Can you work these out from the model? Positions are in its coordinate system, mm. A direction names the side the tool comes from. Round coordinates to 2 decimals unless told otherwise and drop trailing zeros. Loops run counter-clockwise (first coordinate to the right, second up) from the corner with the lowest first, then second, coordinate; pieces in that order, holes last. Notation, with made-up numbers: (-30, 70.25) -> (10, 70.25) arc R18 ccw to (10, 92.25) -> close; hole circle Ø3 at (-30, -24.75). An arc over 180 degrees is marked (long way). Use a Markdown table: item, result.
from build123d import *

# Parameters (mm, degrees)
BOX001_W     = 100
BOX001_H     = 15
BOX001_DEPTH = 4
BOX_W        = 100
BOX_H        = 37
BOX_DEPTH    = 10
FILLET_R     = 1


with BuildPart() as cutter:
    # Box001 → Box001 (new body)
    with BuildSketch(Plane.XY.offset(3)):
        with Locations((50, 7.5)):
            Rectangle(BOX001_W, BOX001_H)
    extrude(amount=BOX001_DEPTH)


with BuildPart() as fillet_body:
    # Box → Box (new body)
    with BuildSketch(Plane.XY):
        with Locations((50, 18.5)):
            Rectangle(BOX_W, BOX_H)
    extrude(amount=BOX_DEPTH)

    # Cut: cut Cutter
    add(cutter.part, mode=Mode.SUBTRACT)

    # Fillet
    fillet_edges = [fillet_body.edges().sort_by_distance(p)[0] for p in [
        (0, 0, 1.5),
        (0, 7.5, 3),
        (0, 15, 5),
        (0, 7.5, 7),
        (0, 0, 8.5),
        (0, 18.5, 10),
        (0, 37, 5),
        (0, 18.5, 0),
        (100, 0, 1.5),
        (50, 0, 3),
        (50, 0, 0),
        (50, 15, 3),
        (100, 7.5, 3),
        (100, 15, 5),
        (50, 15, 7),
        (50, 0, 7),
        (100, 7.5, 7),
        (100, 0, 8.5),
        (50, 0, 10),
        (50, 37, 10),
        (100, 18.5, 10),
        (50, 37, 0),
        (100, 37, 5),
        (100, 18.5, 0),
    ]]
    fillet(fillet_edges, radius=FILLET_R)


solid = fillet_body.part
1. I want a section at A-A (y = 7). Please give me the cut outline in (x, z), plus the area to 3 significant figures.
Answer sheet:
| item | result |
|---|---|
| outline | (0, 1) arc R1 ccw to (1, 0) -> (99, 0) arc R1 ccw to (100, 1) -> (100, 2) arc R1 ccw to (99, 3) -> (1, 3) arc R1 ccw to (0, 2) -> close; (0, 8) arc R1 ccw to (1, 7) -> (99, 7) arc R1 ccw to (100, 8) -> (100, 9) arc R1 ccw to (99, 10) -> (1, 10) arc R1 ccw to (0, 9) -> close |
| area | 598 mm² |
2. I want a section at B-B (x = 56). Please give me the cut outline in (y, z).
Answer sheet:
| item | result |
|---|---|
| outline | (0, 1) arc R1 ccw to (1, 0) -> (36, 0) arc R1 ccw to (37, 1) -> (37, 9) arc R1 ccw to (36, 10) -> (1, 10) arc R1 ccw to (0, 9) -> (0, 8) arc R1 ccw to (1, 7) -> (14, 7) arc R1 cw to (15, 6) -> (15, 4) arc R1 cw to (14, 3) -> (1, 3) arc R1 ccw to (0, 2) -> close |
3. Which directions (+Z, -Z, +X, -X, +Y, -Y) give clear straight access to the entire face, cutting with the end or side of a thin tool? Please do faces 1 (the flat face through (49, 8, 7)), 2 (the flat face through (0, 22, 5)).
Answer sheet:
| item | result |
|---|---|
| face 1 | +X, -X, -Y |
| face 2 | +Z, -Z, -X, +Y, -Y |
4. If we mould it in two halves opening along Z, with no side actions, what happens to faces 3 (the flat face through (49, 37, 5)), 4 (the flat face through (49, 15, 5)), 5 (the flat face through (49, 19, 0))? For each: +Z half, -Z half, draft (parallel to the pull), parting line (faces both ways), or undercut.
Answer sheet:
| item | result |
|---|---|
| face 3 | draft |
| face 4 | undercut |
| face 5 | -Z half |
5. Will this pin go through, and if not, where does the flat tip stop? pin 1 Ø2 at (x, z) = (55, 5.5) entering from -Y.
Answer sheet:
| item | result |
|---|---|
| pin 1 | stops at y = 14.87 |
6. I need wall thicknesses on line 1 (Z direction, x = 30, y = 2); line 2 (Y direction, x = 76, z = 5.75); line 3 (Y direction, x = 15.5, z = 2.75). Which ranges of each line are inside material? Lowest first, please.
Answer sheet:
| item | result |
|---|---|
| line 1 | z = 0 to 3, 7 to 10 |
| line 2 | y = 15 to 37 |
| line 3 | y = 0.34 to 37 |
